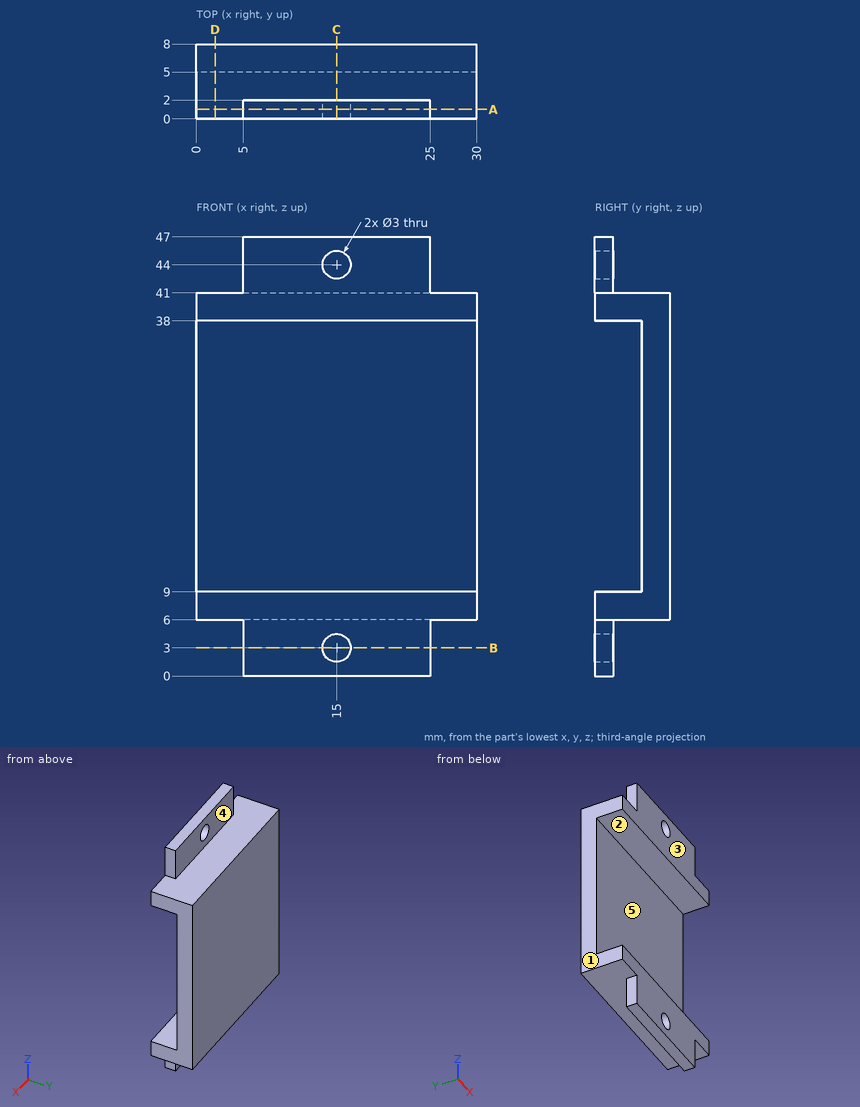
Geometry check sheet. Reference: drawing and pictorial views, mm from the part's lowest x, y, z. A direction names the side the tool comes from. Give positions to 0.01 mm unless a question says otherwise; leave off trailing zeros. Write each loop counter-clockwise with the first axis right and the second up, starting at its lowest first coordinate (ties: lowest second). Pieces come first, ordered by that corner, then holes. Notation, with made-up numbers: (47.5, 8) - (51.5, 8) arc R11 ccw to (51.5, 27) - close; hole circle Ø4 at (19, 85). An arc over 180 degrees is marked (long way). Use a Markdown table: item, result.
Q1. Go/stop test with flat-tipped pins: P1, Ø4, axis at x = 20.5, y = 1.5, coming from the -Z side; P2, Ø1.6, axis at y = 1, z = 2, coming from the -X side; P3, Ø2.5, axis at x = 15, z = 44, coming from the +Y side; P4, Ø1.6, axis at y = 1, z = 44, coming from the +X side. Record where each tip stops, or that it passes through.
Computed:
| item | result |
|---|---|
| P1 | stops at z = 0 |
| P2 | stops at x = 5 |
| P3 | passes through |
| P4 | stops at x = 25 |
Q2. Section check D-D, the plane x = 2. Enter the section's corners in (y, z), then the cut area to 3 significant figures.
Computed:
| item | result |
|---|---|
| outline | (0, 6) - (8, 6) - (8, 41) - (0, 41) - (0, 38) - (5, 38) - (5, 9) - (0, 9) - close |
| area | 135 mm² |
Q3. Draft check along Z on the marked faces 1 and 2. Enter one of: pulls with the +Z half, pulls with the -Z half, needs draft (parallel to the pull), parting line crosses it, or undercut.
Computed:
| item | result |
|---|---|
| face 1 | needs draft |
| face 2 | undercut |
Q4. Set-up check for the marked faces 3, 4 and 5: record each of +Z, -Z, +X, -X, +Y, -Y from which the full face is reachable in a straight line by a thin tool's end or side.
Computed:
| item | result |
|---|---|
| face 3 | +Z, -Z, +X, -X, -Y |
| face 4 | +Z, +X, -X, +Y |
| face 5 | +X, -X, -Y |
Q5. Thickness scan on L1, parallel to Z at x = 15, y = 0.5; L2, parallel to Z at x = 26.25, y = 1; L3, parallel to Z at x = 9.5, y = 1.75. Record the ranges inside material, lowest first. Write a range as [from, to].
Computed:
| item | result |
|---|---|
| L1 | z = [0, 1.5], [4.5, 9], [38, 42.5], [45.5, 47] |
| L2 | z = [6, 9], [38, 41] |
| L3 | z = [0, 9], [38, 47] |
Q6. Section check A-A, the plane y = 1. Enter the section's corners in (x, z), then the cut area to 3 significant figures.
Computed:
| item | result |
|---|---|
| outline | (0, 6) - (5, 6) - (5, 0) - (25, 0) - (25, 6) - (30, 6) - (30, 9) - (0, 9) - close; (0, 38) - (30, 38) - (30, 41) - (25, 41) - (25, 47) - (5, 47) - (5, 41) - (0, 41) - close; hole circle Ø3 at (15, 3); hole circle Ø3 at (15, 44) |
| area | 406 mm² |
Q7. Section check C-C, the plane x = 15. Enter the section's corners in (y, z).
Computed:
| item | result |
|---|---|
| outline | (0, 0) - (2, 0) - (2, 1.5) - (0, 1.5) - close; (0, 4.5) - (2, 4.5) - (2, 6) - (8, 6) - (8, 41) - (2, 41) - (2, 42.5) - (0, 42.5) - (0, 38) - (5, 38) - (5, 9) - (0, 9) - close; (0, 45.5) - (2, 45.5) - (2, 47) - (0, 47) - close |
Q8. Section check B-B, the plane z = 3. Enter the section's corners in (x, y), then the cut area to 3 significant figures.
Computed:
| item | result |
|---|---|
| outline | (5, 0) - (13.5, 0) - (13.5, 2) - (5, 2) - close; (16.5, 0) - (25, 0) - (25, 2) - (16.5, 2) - close |
| area | 34.0 mm² |
